The figure shows three views and two pictorial views of one solid part (mm, origin at its lowest corner). Answer the questions. A direction names the side the tool comes from. Give positions to 0.01 mm unless a question says otherwise; leave off trailing zeros. Order: outer loops, then holes, each group sorted by start corner. A loop starts at its lowest first (then second) coordinate and runs counter-clockwise, first axis right, second up. Notation, with made-up numbers: M 20.5,1 L 28.5,1 A15 ccw 28.5,25 Z; hole C 7,81.5 d3. An arc over 180 degrees is marked long. One line per item, written item: value.
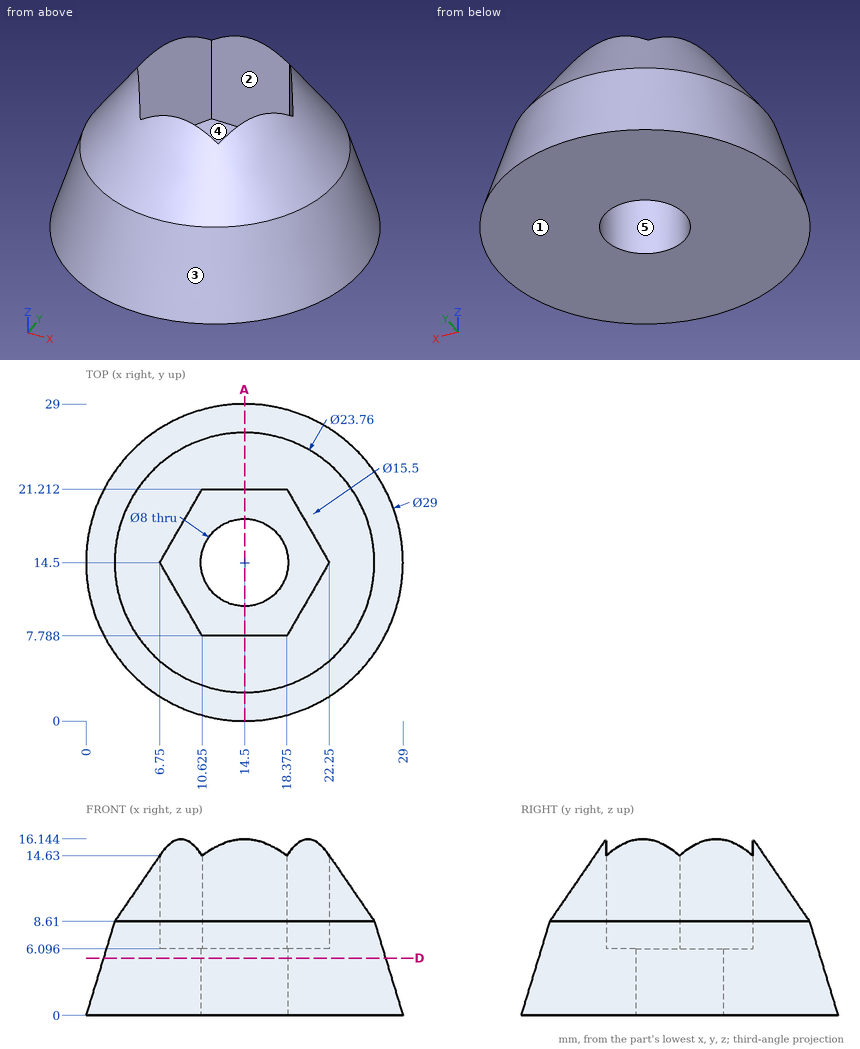
1) Consider probe 1 along Z at (x, y) = (19.25, 15.25); probe 2 along Y at (x, z) = (14.5, 2.5); probe 3 along Y at (x, z) = (8.5, 14.5) (1 decimal). Determine where each line is inside the solid, lowest interval first.
Reported:
probe 1: z = 0 to 6.1
probe 2: y = 0.76 to 10.5, 18.5 to 28.24
probe 3: y = 9.5 to 11.5, 17.5 to 19.5
2) Which of the six approach directions +Z, -Z, +X, -X, +Y, -Y give full straight-line access (tool end or side, diameter ignored) to the marked faces 4 and 5?
Reported:
face 4: +Z
face 5: +Z, -Z
3) Find section D-D, the plane z = 5.25. Write down the section's boundary in (x, y) (1 decimal), plus the area to 3 significant figures.
Reported:
outline: C 14.5,14.5 d25.8; hole C 14.5,14.5 d8
area: 473 mm^2
4) Find section A-A, the plane x = 14.5. Write down the section's boundary in (y, z).
Reported:
outline: M 0,0 L 10.5,0 L 10.5,6.1 L 7.79,6.1 L 7.79,16.14 L 2.62,8.61 Z; M 18.5,0 L 29,0 L 26.38,8.61 L 21.21,16.14 L 21.21,6.1 L 18.5,6.1 Z
5) Each of these flat-tipped pins is pushed along its axis until it touches: pin 1 Ø1 at (y, z) = (24, 7) entering from -X; pin 2 Ø2 at (x, z) = (21, 6) entering from +Y (1 decimal); pin 3 Ø2.5 at (x, z) = (16.5, 10) entering from +Y (1 decimal); pin 4 Ø1.5 at (x, y) = (24, 23) entering from -Z. Where does it stop, or does it pass through?
Reported:
pin 1: stops at x = 5.97
pin 2: stops at y = 26
pin 3: stops at y = 26.1
pin 4: stops at z = 0
6) Determine the mould class of the marked faces 1, 2 and 3 for opening direction X: +X half, -X half, draft (parallel to the pull), parting line (faces both ways), or undercut.
Reported:
face 1: draft
face 2: undercut
face 3: parting line
